Read the model definition and answer for the solid it produces. Units are mm, in the model's axes. A direction names the side the tool comes from. Give positions to 0.01 mm unless a question says otherwise; leave off trailing zeros. Write each loop counter-clockwise with the first axis right and the second up, starting at its lowest first coordinate (ties: lowest second). Pieces come first, ordered by that corner, then holes. Notation, with made-up numbers: M 19.5,72 L 25.5,72 A20 cw 25.5,91 Z; hole C 26.5,27 d11. An arc over 180 degrees is marked long. Write each question's results on one line, items separated by ' | '. Start each with the question number.
```python
from build123d import *

# Parameters (mm, degrees)
F1_DEPTH = 105


with BuildPart() as f1:
    # F0 (on Top) → F1 (new body)
    with BuildSketch(Plane.XY):
        Polygon((-47.451783, 161.583327), (-47.451783, 56.583327), (57.548217, 56.583327), (57.548217, 161.583327), (-44.951783, 161.583327), align=None)
        Polygon((-44.951783, 109.083327), (-44.951783, 158.90345), (55.048217, 158.90345), (55.048217, 58.90345), (-44.951783, 58.90345), align=None, mode=Mode.SUBTRACT)
    extrude(amount=-F1_DEPTH)


solid = f1.part
```
Item 1: Section A-A, the plane y = 116.5 is taken. Determine the outline of the cut face in (x, z).
Item 2: Straight lines are drawn through the part: line 1 (X direction, y = 118, z = -29.5); line 2 (Y direction, x = 30.5, z = -9.5). For each, find the intervals that lie inside material, in ascending order.
Item 3: Section B-B, the plane x = -14 is taken. Determine the outline of the cut face in (y, z).
Item 4: Section C-C, the plane z = -96 is taken. Determine the outline of the cut face in (x, y).
Item 5: Determine the mould class of faces 1 (the flat face through (6, 58.903, -52)), 2 (the flat face through (-44.952, 108, -52)), 3 (the flat face through (4, 56.583, -52)), 4 (the flat face through (-47.452, 110, -52)) for opening direction X: +X half, -X half, draft (parallel to the pull), parting line (faces both ways), or undercut.
Item 6: For faces 5 (the flat face through (-46, 109, -105)), 6 (the flat face through (55.048, 110, -52)), determine the directions among +Z, -Z, +X, -X, +Y, -Y from which every point of the face is accessible in a straight line to the end or side of a thin tool.
Worked out:
1) outline: M -47.45,-105 L -44.95,-105 L -44.95,0 L -47.45,0 Z; M 55.05,-105 L 57.55,-105 L 57.55,0 L 55.05,0 Z
2) line 1: x = -47.45 to -44.95, 55.05 to 57.55 | line 2: y = 56.58 to 58.9, 158.9 to 161.58
3) outline: M 56.58,-105 L 58.9,-105 L 58.9,0 L 56.58,0 Z; M 158.9,-105 L 161.58,-105 L 161.58,0 L 158.9,0 Z
4) outline: M -47.45,56.58 L 57.55,56.58 L 57.55,161.58 L -47.45,161.58 Z; hole M -44.95,58.9 L 55.05,58.9 L 55.05,158.9 L -44.95,158.9 Z
5) face 1: undercut | face 2: undercut | face 3: draft | face 4: -X half
6) face 5: -Z, +X, -X, +Y, -Y | face 6: +Z, -Z
